from build123d import *

# Parameters (mm, degrees)
SKETCH2_W               = 80.518
SKETCH2_H               = 38.9255
BOSS_EXTRUDE1_DEPTH     = 22.987
SKETCH3_W               = 80.518
SKETCH3_H               = 45.974
BOSS_EXTRUDE2_DEPTH     = 11.1125
CHAMFER1_SIZE           = 0.381
SKETCH4_R               = 4.953
CUT_EXTRUDE1_DEPTH      = 28.038
SKETCH5_R               = 3.96875
CUT_EXTRUDE2_DEPTH      = 1.27
CHAMFER2_SIZE           = 0.254
SKETCH6_R               = 3.96875
SKETCH6_R_2             = 3.84175
CUT_EXTRUDE_THIN1_DEPTH = 1.27
CHAMFER3_SIZE           = 0.254
CUT_EXTRUDE3_DEPTH      = 2.032
SKETCH8_R               = 2.75
CUT_EXTRUDE4_DEPTH      = 99.439603917
SKETCH9_R               = 3.556
CUT_EXTRUDE5_DEPTH      = 2.54
SKETCH10_R              = 2.159
CUT_EXTRUDE6_DEPTH      = 4
SKETCH17_R              = 18.19275
BOSS_EXTRUDE4_DEPTH     = 85.217
SKETCH13_R              = 6.858
BOSS_EXTRUDE3_DEPTH     = 2.54
CHAMFER4_SIZE           = 0.762
CUT_EXTRUDE8_DEPTH      = 5.08
SKETCH18_OUTSIDE_W      = 84.27
SKETCH18_OUTSIDE_H      = 88.334
SKETCH18_OUTSIDE_R      = 6.858
CUT_EXTRUDE10_DEPTH     = 2.54
CUT_EXTRUDE11_DEPTH     = 5.08
CHAMFER5_SIZE           = 0.762
CUT_EXTRUDE12_DEPTH     = 10.3124
CUT_EXTRUDE13_START     = 6.35
CUT_EXTRUDE13_DEPTH     = 12.7


with BuildPart() as part:
    # Sketch2 → Boss-Extrude1 (new, symmetric)
    with BuildSketch(Plane.XY):
        with Locations((-41.3385, 19.46275)):
            Rectangle(SKETCH2_W, SKETCH2_H)
    extrude(amount=BOSS_EXTRUDE1_DEPTH, both=True)


with BuildPart() as body_2:
    # Sketch3 → Boss-Extrude2 (new body)
    with BuildSketch(Plane(origin=(0, 38.9255, 0), x_dir=(1, 0, 0), z_dir=(0, 1, 0))):
        with Locations((-41.3385, 0)):
            Rectangle(SKETCH3_W, SKETCH3_H)
    extrude(amount=BOSS_EXTRUDE2_DEPTH)

    # Chamfer1
    chamfer1_edges = [body_2.edges().sort_by_distance(p)[0] for p in [
        (-81.5975, 50.038, 0),
        (-41.3385, 50.038, 22.987),
        (-1.0795, 50.038, 0),
        (-41.3385, 38.9255, 22.987),
        (-81.5975, 38.9255, 0),
        (-41.3385, 38.9255, -22.987),
        (-1.0795, 38.9255, 0),
        (-41.3385, 50.038, -22.987),
    ]]
    chamfer(chamfer1_edges, length=CHAMFER1_SIZE)


with BuildPart() as part_1:
    add(part.part)

    # Combine1: union body 2
    add(body_2.part)

    # Sketch4 → Cut-Extrude1 (cut)
    with BuildSketch(Plane(origin=(0, 50.038, 0), x_dir=(1, 0, 0), z_dir=(0, 1, 0))):
        with Locations(Location((-70.5485, 15.494, 0), (0, 0, 270))):
            Circle(SKETCH4_R)
        with Locations(Location((-30.1625, 16.256, 0), (0, 0, 270))):
            Circle(SKETCH4_R)
        with Locations(Location((-70.5485, -15.494, 0), (0, 0, 270))):
            Circle(SKETCH4_R)
        with Locations(Location((-30.1625, -16.256, 0), (0, 0, 270))):
            Circle(SKETCH4_R)
    extrude(amount=-CUT_EXTRUDE1_DEPTH, mode=Mode.SUBTRACT)

    # Sketch5 → Cut-Extrude2 (cut)
    with BuildSketch(Plane(origin=(0, 50.038, 0), x_dir=(1, 0, 0), z_dir=(0, 1, 0))):
        with Locations(Location((-56.1975, 17.4625, 0), (0, 0, 270))):
            Circle(SKETCH5_R)
        with Locations(Location((-16.51, 17.4625, 0), (0, 0, 270))):
            Circle(SKETCH5_R)
        with Locations(Location((-56.1975, -17.4625, 0), (0, 0, 270))):
            Circle(SKETCH5_R)
        with Locations(Location((-16.51, -17.4625, 0), (0, 0, 270))):
            Circle(SKETCH5_R)
    extrude(amount=-CUT_EXTRUDE2_DEPTH, mode=Mode.SUBTRACT)

    # Chamfer2
    chamfer2_edges = [part_1.edges().sort_by_distance(p)[0] for p in [
        (-70.5485, 50.038, -20.447),
        (-30.1625, 50.038, -21.209),
        (-70.5485, 50.038, 10.541),
        (-30.1625, 50.038, 11.303),
        (-56.1975, 50.038, -21.43125),
        (-16.51, 50.038, -21.43125),
        (-56.1975, 50.038, 13.49375),
        (-16.51, 50.038, 13.49375),
    ]]
    chamfer(chamfer2_edges, length=CHAMFER2_SIZE)

    # Sketch6 → Cut-Extrude-Thin1 (cut)
    # profile 1 of 4: a face of its own
    with BuildSketch(Plane(origin=(0, 48.768, 0), x_dir=(1, 0, 0), z_dir=(0, 1, 0))):
        with Locations((-56.1975, 17.4625)):
            Circle(SKETCH6_R)
        with Locations((-56.1975, 17.4625)):
            Circle(SKETCH6_R_2, mode=Mode.SUBTRACT)
    # profile 2 of 4: a face of its own
    with BuildSketch(Plane(origin=(0, 48.768, 0), x_dir=(1, 0, 0), z_dir=(0, 1, 0))):
        with Locations((-16.51, 17.4625)):
            Circle(SKETCH6_R)
        with Locations((-16.51, 17.4625)):
            Circle(SKETCH6_R_2, mode=Mode.SUBTRACT)
    # profile 3 of 4: a face of its own
    with BuildSketch(Plane(origin=(0, 48.768, 0), x_dir=(1, 0, 0), z_dir=(0, 1, 0))):
        with Locations((-16.51, -17.4625)):
            Circle(SKETCH6_R)
        with Locations((-16.51, -17.4625)):
            Circle(SKETCH6_R_2, mode=Mode.SUBTRACT)
    # profile 4 of 4: a face of its own
    with BuildSketch(Plane(origin=(0, 48.768, 0), x_dir=(1, 0, 0), z_dir=(0, 1, 0))):
        with Locations((-56.1975, -17.4625)):
            Circle(SKETCH6_R)
        with Locations((-56.1975, -17.4625)):
            Circle(SKETCH6_R_2, mode=Mode.SUBTRACT)
    extrude(amount=-CUT_EXTRUDE_THIN1_DEPTH, mode=Mode.SUBTRACT)

    # Chamfer3
    chamfer3_edges = [part_1.edges().sort_by_distance(p)[0] for p in [
        (-20.35175, 48.768, -17.4625),
        (-20.35175, 48.768, 17.4625),
        (-60.03925, 48.768, 17.4625),
        (-60.03925, 48.768, -17.4625),
    ]]
    chamfer(chamfer3_edges, length=CHAMFER3_SIZE)

    # Sketch7 → Cut-Extrude3 (cut)
    with BuildSketch(Plane(origin=(0, 48.768, 0), x_dir=(1, 0, 0), z_dir=(0, 1, 0))):
        Polygon((-56.1975, 19.750192707), (-58.1787, 18.606346353), (-58.1787, 16.318653647), (-56.1975, 15.174807293), (-54.2163, 16.318653647), (-54.2163, 18.606346353), align=None)
        Polygon((-56.1975, -15.174807293), (-58.1787, -16.318653647), (-58.1787, -18.606346353), (-56.1975, -19.750192707), (-54.2163, -18.606346353), (-54.2163, -16.318653647), align=None)
        Polygon((-16.51, -14.958811275), (-18.678258039, -16.210655638), (-18.678258039, -18.714344362), (-16.51, -19.966188725), (-14.341741961, -18.714344362), (-14.341741961, -16.210655638), align=None)
        Polygon((-16.51, 19.966188725), (-18.678258039, 18.714344362), (-18.678258039, 16.210655638), (-16.51, 14.958811275), (-14.341741961, 16.210655638), (-14.341741961, 18.714344362), align=None)
    extrude(amount=-CUT_EXTRUDE3_DEPTH, mode=Mode.SUBTRACT)

    # Sketch8 → Cut-Extrude4 (cut, through all)
    with BuildSketch(Plane(origin=(0, 50.038, 0), x_dir=(1, 0, 0), z_dir=(0, 1, 0))):
        with Locations(Location((-70.5485, 15.494, 0), (0, 0, 270))):
            Circle(SKETCH8_R)
        with Locations(Location((-30.1625, 16.256, 0), (0, 0, 270))):
            Circle(SKETCH8_R)
        with Locations(Location((-30.1625, -16.256, 0), (0, 0, 270))):
            Circle(SKETCH8_R)
        with Locations(Location((-70.5485, -15.494, 0), (0, 0, 270))):
            Circle(SKETCH8_R)
    extrude(amount=-CUT_EXTRUDE4_DEPTH, mode=Mode.SUBTRACT)

    # Sketch9 → Cut-Extrude5 (cut)
    with BuildSketch(Plane.XZ):
        with Locations(Location((-48.9585, 10.414, 0), (0, 0, 270))):
            Circle(SKETCH9_R)
        with Locations(Location((-48.9585, -10.414, 0), (0, 0, 270))):
            Circle(SKETCH9_R)
        with Locations(Location((-57.8485, 0, 0), (0, 0, 270))):
            Circle(SKETCH9_R)
        with Locations(Location((-40.3225, 0, 0), (0, 0, 270))):
            Circle(SKETCH9_R)
    extrude(amount=-CUT_EXTRUDE5_DEPTH, mode=Mode.SUBTRACT)

    # Sketch10 → Cut-Extrude6 (cut)
    with BuildSketch(Plane.XZ):
        with Locations(Location((-37.5285, 15.494, 0), (0, 0, 270))):
            Circle(SKETCH10_R)
    extrude(amount=-CUT_EXTRUDE6_DEPTH, mode=Mode.SUBTRACT)

    # Cut-Extrude7 cone 1 section (through the dimple's axis) → Cut-Extrude7 (revolve, cut)
    with BuildSketch(Plane(origin=(-48.9585, 2.54, 10.414), x_dir=(0, 0, -1), z_dir=(1, 0, 0))):
        Polygon((0, 0), (3.556, 0), (0, 3.556), align=None)
    revolve(axis=Axis((-48.9585, 2.54, 10.414), (0, 1, 0)), mode=Mode.SUBTRACT)

    # Cut-Extrude7 cone 2 section (through the dimple's axis) → Cut-Extrude7 cone 2 (revolve, cut)
    with BuildSketch(Plane(origin=(-40.3225, 2.54, 0), x_dir=(0, 0, -1), z_dir=(1, 0, 0))):
        Polygon((0, 0), (3.556, 0), (0, 3.556), align=None)
    revolve(axis=Axis((-40.3225, 2.54, 0), (0, 1, 0)), mode=Mode.SUBTRACT)

    # Cut-Extrude7 cone 3 section (through the dimple's axis) → Cut-Extrude7 cone 3 (revolve, cut)
    with BuildSketch(Plane(origin=(-57.8485, 2.54, 0), x_dir=(0, 0, -1), z_dir=(1, 0, 0))):
        Polygon((0, 0), (3.556, 0), (0, 3.556), align=None)
    revolve(axis=Axis((-57.8485, 2.54, 0), (0, 1, 0)), mode=Mode.SUBTRACT)

    # Cut-Extrude7 cone 4 section (through the dimple's axis) → Cut-Extrude7 cone 4 (revolve, cut)
    with BuildSketch(Plane(origin=(-48.9585, 2.54, -10.414), x_dir=(0, 0, -1), z_dir=(1, 0, 0))):
        Polygon((0, 0), (3.556, 0), (0, 3.556), align=None)
    revolve(axis=Axis((-48.9585, 2.54, -10.414), (0, 1, 0)), mode=Mode.SUBTRACT)

    # Sketch17 → Boss-Extrude4 (add)
    with BuildSketch(Plane(origin=(-1.0795, 0, 0), x_dir=(0, 0, -1), z_dir=(1, 0, 0))):
        with Locations(Location((0, 19.46275, 0), (0, 0, 180))):
            Circle(SKETCH17_R)
    extrude(amount=BOSS_EXTRUDE4_DEPTH)

    # Sketch13 → Boss-Extrude3 (add)
    with BuildSketch(Plane.ZY.offset(81.5975)):
        with Locations(Location((0, 19.46275, 0), (0, 0, 180))):
            Circle(SKETCH13_R)
    extrude(amount=BOSS_EXTRUDE3_DEPTH)

    # Chamfer4
    chamfer4_edges = [part_1.edges().sort_by_distance(p)[0] for p in [
        (-84.1375, 19.46275, 6.858),
    ]]
    chamfer(chamfer4_edges, length=CHAMFER4_SIZE)

    # Sketch14 → Cut-Extrude8 (cut)
    with BuildSketch(Plane.ZY.offset(84.1375)):
        Polygon((0, 23.128924209), (-3.175, 21.295837105), (-3.175, 17.629662895), (0, 15.796575791), (3.175, 17.629662895), (3.175, 21.295837105), align=None)
    extrude(amount=-CUT_EXTRUDE8_DEPTH, mode=Mode.SUBTRACT)

    # Cut-Extrude9 cone 1 section (through the dimple's axis) → Cut-Extrude9 (revolve, cut)
    with BuildSketch(Plane(origin=(-84.1375, 19.46275, 0), x_dir=(0, 0, 1), z_dir=(0, 1, 0))):
        Polygon((0, 0), (3.666174209, 0), (0, 3.666174209), align=None)
    revolve(axis=Axis((-84.1375, 19.46275, 0), (1, 0, 0)), mode=Mode.SUBTRACT)

    # Sketch18 outside → Cut-Extrude10 (cut)
    with BuildSketch(Plane(origin=(84.1375, 0, 0), x_dir=(0, 0, -1), z_dir=(1, 0, 0))):
        with Locations((0, 25.019)):
            Rectangle(SKETCH18_OUTSIDE_W, SKETCH18_OUTSIDE_H)
        with Locations((0, 19.46275)):
            Circle(SKETCH18_OUTSIDE_R, mode=Mode.SUBTRACT)
    extrude(amount=-CUT_EXTRUDE10_DEPTH, mode=Mode.SUBTRACT)

    # Sketch19 → Cut-Extrude11 (cut)
    with BuildSketch(Plane(origin=(84.1375, 0, 0), x_dir=(0, 0, -1), z_dir=(1, 0, 0))):
        Polygon((3.175, 21.295837105), (0, 23.128924209), (-3.175, 21.295837105), (-3.175, 17.629662895), (0, 15.796575791), (3.175, 17.629662895), align=None)
    extrude(amount=-CUT_EXTRUDE11_DEPTH, mode=Mode.SUBTRACT)

    # Chamfer5
    chamfer5_edges = [part_1.edges().sort_by_distance(p)[0] for p in [
        (84.1375, 19.46275, 6.858),
    ]]
    chamfer(chamfer5_edges, length=CHAMFER5_SIZE)

    # Sketch20 → Cut-Revolve1 (revolve, cut)
    with BuildSketch(Plane.XY, mode=Mode.PRIVATE) as cut_revolve1_sk:
        Polygon((81.5975, 32.9565), (78.4225, 33.807238686), (67.31, 33.807238686), (67.31, 36.804761314), (64.135, 37.6555), (60.1726, 37.6555), (60.1726, 37.1475), (59.6646, 37.1475), (59.6646, 40.8305), (81.5975, 40.8305), align=None)
    revolve(cut_revolve1_sk.sketch.rotate(Axis((83.3755, 19.46275, 0), (-1, 0, 0)), 90), axis=Axis((83.3755, 19.46275, 0), (-1, 0, 0)), mode=Mode.SUBTRACT)

    # Sketch21 → Cut-Extrude12 (cut)
    with BuildSketch(Plane(origin=(67.31, 0, 0), x_dir=(0, 0, -1), z_dir=(1, 0, 0))):
        with BuildLine():
            Line((8.000347905, 7.5565), (-8.000347905, 7.5565))
            ThreePointArc((-8.000347905, 7.5565), (0, 5.118261314), (8.000347905, 7.5565))
        make_face()
        with BuildLine():
            Line((-8.000347905, 31.369), (8.000347905, 31.369))
            ThreePointArc((8.000347905, 31.369), (0, 33.807238686), (-8.000347905, 31.369))
        make_face()
    extrude(amount=CUT_EXTRUDE12_DEPTH, mode=Mode.SUBTRACT)

    # Sketch22 → Cut-Extrude13 (cut)
    with BuildSketch(Plane(origin=(-1.0795, 0, 0), x_dir=(0, 0, -1), z_dir=(1, 0, 0)).offset(CUT_EXTRUDE13_START)):
        with BuildLine():
            Line((-15.875, 28.348723642), (-15.875, 10.576776358))
            ThreePointArc((-15.875, 10.576776358), (-18.19275, 19.46275), (-15.875, 28.348723642))
        make_face()
        with BuildLine():
            Line((15.875, 28.348723642), (15.875, 10.576776358))
            ThreePointArc((15.875, 10.576776358), (18.19275, 19.46275), (15.875, 28.348723642))
        make_face()
    extrude(amount=CUT_EXTRUDE13_DEPTH, mode=Mode.SUBTRACT)


solid = part_1.part
Input: part model. Units: mm. Frame: model coordinates. A direction names the side the tool comes from. Coordinates: 2 decimals unless noted, no trailing zeros. Loops run counter-clockwise (first coordinate to the right, second up) from the corner with the lowest first, then second, coordinate; pieces in that order, holes last. Notation, with made-up numbers: (78.5, 45.5) - (117.5, 45.5) arc R33 cw to (117.5, 75.5) - close; hole circle Ø9 at (-31, 69). An arc over 180 degrees is marked (long way). Answer in a Markdown table with one row per item. Add a question column.
Item 1: Mould query, pull axis Y, two halves, no side actions, for faces 4 (the conical face through (81.399, 32.688, 2.937)), 5 (the conical face through (-56.909, 5.133, 0.209)), 6 (the flat face through (-81.633, 16.7, 1.565)), 7 (the flat face through (81.633, 16.7, -1.565)). Classes: released by +Y, released by -Y, zero draft, split by the parting line, or undercut.
Item 2: Contact query for flat-ended pins moving along their axis: P1, Ø8.5, axis at y = 44.5, z = -4.5, coming from the +X side; P2, Ø1.3, axis at x = -16, z = 18, coming from the +Y side; P3, Ø3, axis at x = 25, z = -14, coming from the +Y side. Output: stop coordinate, or through.
Item 3: Section query B-B on x = 8.5. Return the cut outline in (y, z) (1 decimal), then the cut area to 3 significant figures.
Item 4: Access query for faces 1 (the flat face through (12, 20, 15.875)), 2 (the cylindrical face through (28.867, 18.663, -18.175)), 3 (the flat face through (-56, 46.736, 17)). Directions: +Z, -Z, +X, -X, +Y, -Y. A direction counts if a zero-diameter tool reaches every point of the face in a straight line with its end or side. Return the directions, or none.
Item 5: Line query: line 1 along X through (y, z) = (24.5, -15); line 2 along X through (y, z) = (23.5, 12.5); line 3 along X through (y, z) = (16.5, -16.5). Output: solid intervals per line, ascending. Write a range as [from, to].
Item 6: Section query A-A on y = 43.5. Return the cut outline in (x, z), then the cut area to 3 significant figures.
Recorded:
| question | item | result |
|---|---|---|
| 1 | face 4 | split by the parting line |
| 1 | face 5 | released by -Y |
| 1 | face 6 | undercut |
| 1 | face 7 | undercut |
| 2 | P1 | x = -1.08 |
| 2 | P2 | y = 46.74 |
| 2 | P3 | y = 32.68 |
| 3 | outline | (10.6, -15.9) - (28.3, -15.9) arc R18.2 ccw to (28.3, 15.9) - (10.6, 15.9) arc R18.2 ccw to start |
| 3 | area | 984 mm^2 |
| 4 | face 1 | +Z, +Y, -Y |
| 4 | face 2 | +X |
| 4 | face 3 | +Y |
| 5 | line 1 | [-81.6, -75.48], [-65.62, -34.95], [-25.37, 67.31] |
| 5 | line 2 | [-81.6, -74.49], [-66.6, -33.39], [-26.93, 81.6] |
| 5 | line 3 | [-81.6, -73.11], [-67.99, -32.9], [-27.42, 5.27], [17.97, 67.31] |
| 6 | outline | (-81.6, -22.99) - (-1.08, -22.99) - (-1.08, 22.99) - (-81.6, 22.99) - close; hole circle Ø9.91 at (-70.55, -15.49); hole circle Ø9.91 at (-70.55, 15.49); hole circle Ø9.91 at (-30.16, -16.26); hole circle Ø9.91 at (-30.16, 16.26) |
| 6 | area | 3,390 mm^2 |
